from build123d import *

# Parameters (mm, degrees)
SKETCH1_R           = 5.42927296
SKETCH1_R_2         = 18.05
SKETCH1_R_3         = 3
BOSS_EXTRUDE1_DEPTH = 6.2


with BuildPart() as part:
    # Sketch1 → Boss-Extrude1 (new body)
    with BuildSketch(Plane.XY):
        with BuildLine():
            ThreePointArc((22.30856743, 80.228990984), (19.658905911, 82.429667946), (16.30856743, 83.228990984))
            ThreePointArc((16.30856743, 83.228990984), (-10.777239886, 80.224067192), (-37.702247141, 76.015206396))
            Line((-37.702247141, 76.015206396), (-37.971821537, 75.970473087))
            Line((-37.971821537, 75.970473087), (-68.682554074, 70.874318891))
            ThreePointArc((-68.682554074, 70.874318891), (-75.78826802, 66.335898634), (-77.417928756, 58.063496625))
            Line((-77.417928756, 58.063496625), (-72.629383419, 35.535152501))
            Line((-72.629383419, 35.535152501), (-73.507041371, 35.028436446))
            ThreePointArc((-73.507041371, 35.028436446), (-77.979929304, 29.199255403), (-77.020885248, 21.91459257))
            Line((-77.020885248, 21.91459257), (-66.455316905, 3.61449139))
            ThreePointArc((-66.455316905, 3.61449139), (-65.048189041, -4.003273118), (-62.651846579, -11.369947247))
            Line((-62.651846579, -11.369947247), (-53.06582932, -52.891535091))
            Line((-53.06582932, -52.891535091), (-53.055513447, -82.591545802))
            Line((-53.055513447, -82.591545802), (78.944486553, -82.591545802))
            Line((78.944486553, -82.591545802), (78.944486553, -50.191545802))
            Line((78.944486553, -50.191545802), (78.944486553, 1.408454198))
            ThreePointArc((78.944486553, 1.408454198), (53.936647448, 43.197185389), (22.30856743, 80.228990984))
        make_face()
        with Locations(Location((-66.592661175, 60.23811882, 0), (0, 0, 180))):
            Circle(SKETCH1_R, mode=Mode.SUBTRACT)
        with Locations(Location((-19.455513478, 30.208443842, 0), (0, 0, 180))):
            Circle(SKETCH1_R_2, mode=Mode.SUBTRACT)
        with Locations(Location((8.19601445, 71.114592564, 0), (0, 0, 180))):
            Circle(SKETCH1_R_3, mode=Mode.SUBTRACT)
        with Locations(Location((-24.307041406, -50.188463292, 0), (0, 0, 180))):
            Circle(SKETCH1_R_3, mode=Mode.SUBTRACT)
        with Locations(Location((-68.707041371, 26.71459257, 0), (0, 0, 180))):
            Circle(SKETCH1_R_3, mode=Mode.SUBTRACT)
        with Locations(Location((52.59601445, -5.788463292, 0), (0, 0, 180))):
            Circle(SKETCH1_R_3, mode=Mode.SUBTRACT)
        with BuildLine():
            ThreePointArc((22.931673418, -46.402822526), (20.150851995, -53.151619974), (25.944486522, -57.591556206))
            Line((25.944486522, -57.591556206), (56.944486522, -57.591556206))
            ThreePointArc((56.944486522, -57.591556206), (61.18712721, -55.834196893), (62.944486522, -51.591556206))
            Line((62.944486522, -51.591556206), (62.944486522, -33.591556206))
            ThreePointArc((62.944486522, -33.591556206), (59.938073115, -28.391706274), (53.931673418, -28.402822526))
            Line((53.931673418, -28.402822526), (22.931673418, -46.402822526))
        make_face(mode=Mode.SUBTRACT)
    extrude(amount=BOSS_EXTRUDE1_DEPTH)


solid = part.part
Model file for the job. Use its own axes, mm. A direction names the side the tool comes from. Give positions to 0.01 mm unless a question says otherwise; leave off trailing zeros. Write each loop counter-clockwise with the first axis right and the second up, starting at its lowest first coordinate (ties: lowest second). Pieces come first, ordered by that corner, then holes. Notation, with made-up numbers: M 44.5,-16 L 101.5,-16 A14 ccw 101.5,10 Z; hole C 65,9.5 d7. An arc over 180 degrees is marked long. One line per item, written item: value. Start each with the question number.
Q1. Saw through at C-C, the plane y = -36. Write the cut outline in (x, z), plus the area to 3 significant figures.
Q2. Two-plate mould, pull along X, no slides. Class faces 4 (the flat face through (-1, 1, 0)), 5 (the cylindrical face through (-77.952, 29.301, 3.057)), 6 (the cylindrical face through (-65.42, 65.54, 3.06)): +X half, -X half, draft (parallel to the pull), parting line (faces both ways), or undercut.
Q3. Saw through at A-A, the plane x = 51.5. Write the cut outline in (y, z), plus the area to 3 significant figures.
Q4. Probe probe 1 along Y at (x, z) = (-25, 1.5); probe 2 along X at (y, z) = (26.5, 5.5); probe 3 along Y at (x, z) = (-27, 6). List the from-to ranges inside material, lowest first. Write a range as [from, to].
Q5. Drop flat-ended pins along their axis: pin 1 Ø1.5 at (x, z) = (-53, 2) entering from +Y; pin 2 Ø2 at (y, z) = (58.5, 2) entering from +X; pin 3 Ø1 at (y, z) = (8.5, 2) entering from -X. Give the stop position or say it passes through.
Q6. Saw through at D-D, the plane z = 2.5. Write the cut outline in (x, y), plus the area to 3 significant figures.
Q7. Saw through at B-B, the plane x = -33. Write the cut outline in (y, z).
Q8. 3-axis set-ups, long thin cutter, end or side, ignore diameter. For faces 1 (the flat face through (78.944, -41, 3)), 2 (the flat face through (-75.057, 46.957, 3.057)), 3 (the flat face through (41, -57.592, 3)): which of +Z, -Z, +X, -X, +Y, -Y reach the whole face in a straight line?
Output values:
1. outline: M -56.97,0 L 40.85,0 L 40.85,6.2 L -56.97,6.2 Z; M 62.94,0 L 78.94,0 L 78.94,6.2 L 62.94,6.2 Z
1. area: 706 mm²
2. face 4: draft
2. face 5: -X half
2. face 6: undercut
3. outline: M -82.59,0 L -57.59,0 L -57.59,6.2 L -82.59,6.2 Z; M -29.81,0 L -8.58,0 L -8.58,6.2 L -29.81,6.2 Z; M -3,0 L 46.54,0 L 46.54,6.2 L -3,6.2 Z
3. area: 594 mm²
4. probe 1: y = [-82.59, -53.11], [-47.27, 13.03], [47.39, 78.15]
4. probe 2: x = [-78.3, -71.7], [-65.71, -37.12], [-1.79, 65.08]
4. probe 3: y = [-82.59, -51.51], [-48.87, 13.81], [46.61, 77.84]
5. pin 1: stops at y = 73.6
5. pin 2: stops at x = 42.97
5. pin 3: stops at x = -69.56
6. outline: M -77.42,58.06 L -72.63,35.54 L -73.51,35.03 A9.6 ccw -77.02,21.91 L -66.46,3.61 A58.8 ccw -62.65,-11.37 L -53.07,-52.89 L -53.06,-82.59 L 78.94,-82.59 L 78.94,1.41 A290.93 ccw 22.31,80.23 A7.57 ccw 16.31,83.23 A611.44 ccw -37.7,76.02 L -68.68,70.87 A10.73 ccw Z; hole C -66.59,60.24 d10.86; hole C -68.71,26.71 d6; hole C -19.46,30.21 d36.1; hole C -24.31,-50.19 d6; hole C 8.2,71.11 d6; hole M 22.93,-46.4 A6 ccw 25.94,-57.59 L 56.94,-57.59 A6 ccw 62.94,-51.59 L 62.94,-33.59 A6 ccw 53.93,-28.4 Z; hole C 52.6,-5.79 d6
6. area: 19,200 mm²
7. outline: M -82.59,0 L 18.28,0 L 18.28,6.2 L -82.59,6.2 Z; M 42.14,0 L 76.84,0 L 76.84,6.2 L 42.14,6.2 Z
8. face 1: +Z, -Z, +X, +Y, -Y
8. face 2: +Z, -Z, -X
8. face 3: +Z, -Z
